Verification items for the finished model (mm, model axes). Coordinates: 2 decimals unless noted, no trailing zeros. Order: outer loops, then holes, each group sorted by start corner. A loop starts at its lowest first (then second) coordinate and runs counter-clockwise, first axis right, second up. Notation, with made-up numbers: M 60,-6 L 95,-6 A18 ccw 95,29 Z; hole C -31,83.25 d2. An arc over 180 degrees is marked long. Return JSON: item names as keys, results as strings. Group by question number.
1. Gauge pin test, flat ends, axial feed: pin 1 (2.5 mm diameter, centred on x = 85.5, z = 2, fed in from +Y); pin 2 (5 mm diameter, centred on x = 62.5, y = 2, fed in from +Z). Record the tip position at first contact, or that the pin passes through.
2. Material ranges on line 1 along Y through (x, z) = (-80, 3.8); line 2 along Y through (x, z) = (11.5, 3); line 3 along X through (y, z) = (-0.5, 2.85), recorded low to high.
3. Section check A-A, the plane y = 3.5. Give the number of separate pieces and of enclosed holes in the cut face, plus the area to 3 significant figures.
4. Section check C-C, the plane x = -76.5. Record the cut outline in (y, z).
```python
from build123d import *

# Parameters (mm, degrees)
SKETCH1_W           = 304.8
SKETCH1_H           = 12.7
BOSS_EXTRUDE1_DEPTH = 5.08
CUT_EXTRUDE1_DEPTH  = 153.616804121


with BuildPart() as part:
    # Sketch1 → Boss-Extrude1 (new body)
    with BuildSketch(Plane.XY):
        Rectangle(SKETCH1_W, SKETCH1_H)
    extrude(amount=BOSS_EXTRUDE1_DEPTH)

    # Sketch2 → Cut-Extrude1 (cut, through all)
    with BuildSketch(Plane.XY.offset(5.08)):
        Polygon((115.686465089, 0), (128.386465089, 0), (133.714747747, 6.35), (110.358182431, 6.35), align=None)
        Polygon((149.203030405, 0), (152.4, 0), (152.4, 6.35), (143.874747747, 6.35), align=None)
        Polygon((149.203030405, 0), (152.4, -3.81), (152.4, 0), align=None)
        Polygon((152.4, -3.81), (147.32, -6.35), (152.4, -6.35), align=None)
        Polygon((82.169899773, 0), (94.869899773, 0), (100.198182431, 6.35), (76.841617115, 6.35), align=None)
        Polygon((48.653334457, 0), (61.353334457, 0), (66.681617115, 6.35), (43.325051799, 6.35), align=None)
        Polygon((9.808486483, 6.35), (15.136769141, 0), (27.836769141, 0), (33.165051799, 6.35), align=None)
        Polygon((-23.708078833, 6.35), (-18.379796175, 0), (-5.679796175, 0), (-0.351513517, 6.35), align=None)
        Polygon((-57.224644148, 6.35), (-51.89636149, 0), (-39.19636149, 0), (-33.868078833, 6.35), align=None)
        Polygon((-90.741209464, 6.35), (-85.412926806, 0), (-72.712926806, 0), (-67.384644148, 6.35), align=None)
    extrude(amount=-CUT_EXTRUDE1_DEPTH, mode=Mode.SUBTRACT)


solid = part.part
```
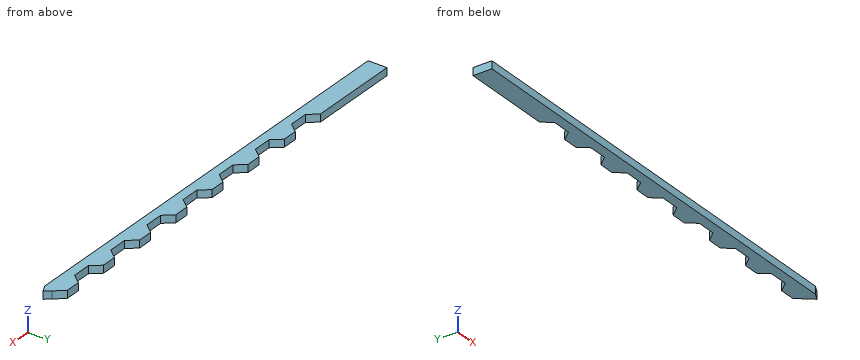
Answers follow:
{
 "1": {"pin 1": "y = 0", "pin 2": "z = 5.08"},
 "2": {"line 1": "-6.35 to 0", "line 2": "-6.35 to 4.33", "line 3": "-152.4 to 149.62"},
 "3": {"separate pieces": "8", "enclosed holes": "0", "area": "857 mm^2"},
 "4": {"outline": "M -6.35,0 L 0,0 L 0,5.08 L -6.35,5.08 Z"}
}
